Autodesk Inventor part; units mm, degrees
ref_plane "YZ Plane" through (0, 0, 0) normal (1, 0, 0) x (0, 1, 0)
ref_plane "XZ Plane" through (0, 0, 0) normal (0, 1, 0) x (-1, 0, 0)
ref_plane "XY Plane" through (0, 0, 0) normal (0, 0, 1) x (1, 0, 0)
sketch "Sketch1" plane through (0, 0, 0) normal (0, 0, 1) x (1, 0, 0)
  line L0 (-750, -950) -> (750, -950)
  line L1 (750, -950) -> (750, 950)
  line L2 (750, 950) -> (-750, 950)
  line L3 (-750, 950) -> (-750, -950)
  line L4 (-750, -950) -> (750, 950) construction
  line L5 (750, -950) -> (-750, 950) construction
  point P0 (0, 0)
  dimension "d0" = 1500
  dimension "d1" = 1900
extrude "Plate1" add sketch "Sketch1" along normal blind 3
sketch "Sketch2" plane through (750, 947.8787, 0.8787) normal (0, 0.7071068, 0.7071068) x (-1, 0, 0)
  line L0 (1500, 0) -> (0, 0)
  line L1 (0, 0) -> (0, -212)
  line L2 (0, -212) -> (1500, -212)
  line L3 (1500, -212) -> (1500, 0)
edge flange "Flange1" height 212 angle 45 thickness 3 bend radius 5 thickness toward (0, 0.7071068, 0.7071068) relief round relief width 3 relief depth 1.5 corner gap 5 corner form 0 edges at (0, 950, 0) (0, -950, 0) wall of the first edge with corners at (-750, 947.8787, 0.8787) (750, 947.8787, 0.8787) (750, 1097.7853, -149.028) (-750, 1097.7853, -149.028)
bend "Bend1"
corner "Corner1"
equation "\"d2\" = Thickness"
equation "\"d3\" = BendReliefWidth"
equation "\"d4\" = BendReliefDepth"
equation "\"d5\" = MinimumRemnant"
equation "\"d6\" = TransitionRadius"
equation "\"d9\" = BendRadius"
equation "\"d10\" = CornerReliefSize"
equation "\"d11\" = GapSize"
equation "\"d12\" = JacobiRadiusSize"
equation "\"BendReliefWidth\" = Thickness"
equation "\"BendReliefDepth\" = 0.5 * Thickness"
equation "\"CornerReliefSize\" = 4 * Thickness"
equation "\"MinimumRemnant\" = 2 * Thickness"
equation "\"TransitionRadius\" = BendRadius"
equation "\"JacobiRadiusSize\" = BendRadius"
equation "\"GapSize\" = Thickness"
properties part number "BSH 010 floor 1" material "09g2s"
Check sheet for the modelled part. Datum: model origin and axes. Units: mm. Give positions to 0.01 mm unless a question says otherwise; leave off trailing zeros. Write each loop counter-clockwise with the first axis right and the second up, starting at its lowest first coordinate (ties: lowest second). Pieces come first, ordered by that corner, then holes. Notation, with made-up numbers: M -19,50.5 L 24,50.5 A19 ccw 24,72.5 Z; hole C 37.5,-33 d8. An arc over 180 degrees is marked long. Use one line per item in the form item = value.
(1) Draft check along Y on faces 1 (the flat face through (-10, 13, 3)), 2 (the flat face through (-10, 13, 0)), 3 (the flat face through (10, 1027, -74)), 4 (the flat face through (-10, -1027, -74)). Enter one of: pulls with the +Y half, pulls with the -Y half, needs draft (parallel to the pull), parting line crosses it, or undercut.
Answer block:
face_1 = needs draft
face_2 = undercut
face_3 = pulls with the +Y half
face_4 = pulls with the -Y half
(2) Section check A-A on z = -69. Record the boundary of the cut face in (x, y).
Answer block:
outline = M -750,-1022 L 750,-1022 L 750,-1017.76 L -750,-1017.76 Z; M -750,1017.76 L 750,1017.76 L 750,1022 L -750,1022 Z
(3) Section check B-B on x = -194. Record the boundary of the cut face in (y, z), plus the area to 3 significant figures.
Answer block:
outline = M -1099.91,-146.91 L -1097.79,-149.03 L -950.22,-1.46 A5 cw -946.69,0 L 946.69,0 A5 cw 950.22,-1.46 L 1097.79,-149.03 L 1099.91,-146.91 L 952.34,0.66 A8 ccw 946.69,3 L -946.69,3 A8 ccw -952.34,0.66 Z
area = 6,960 mm2
(4) Depth check by flat-ended pin: P1, Ø3, axis at x = -335, z = -84, coming from the +Y side; P2, Ø10, axis at x = 8.5, z = -63.5, coming from the -Y side; P3, Ø6, axis at x = 511.5, z = -21.5, coming from the -Y side. Enter the tip coordinate at first touch or a pass-through.
Answer block:
P1 = 1038.5
P2 = -1021.5
P3 = -977.5
(5) Material ranges on line 1 along Z through (x, y) = (-611, 429); line 2 along Y through (x, z) = (317, -22.5); line 3 along Y through (x, z) = (-190, -46), recorded low to high.
Answer block:
line_1 = 0 to 3
line_2 = -975.5 to -971.26, 971.26 to 975.5
line_3 = -999 to -994.76, 994.76 to 999
(6) Section check C-C on y = -559. Record the boundary of the cut face in (x, z), plus the area to 3 significant figures.
Answer block:
outline = M -750,0 L 750,0 L 750,3 L -750,3 Z
area = 4,500 mm2
